```python
from build123d import *

# Parameters (mm, degrees)
SKETCH2_W               = 26
SKETCH2_H               = 26
BOSS_EXTRUDE1_DEPTH     = 53
CUT_EXTRUDE2_DEPTH      = 1
CUT_EXTRUDE2_DEPTH_BACK = 54
SKETCH4_W               = 11
SKETCH4_H               = 5
CUT_EXTRUDE3_DEPTH      = 27
SKETCH5_W               = 17
SKETCH5_H               = 17
CUT_EXTRUDE4_DEPTH      = 21.226470685
BOSS_EXTRUDE3_DEPTH     = 7
BOSS_EXTRUDE4_DEPTH     = 7


with BuildPart() as part:
    # Sketch2 → Boss-Extrude1 (new body)
    with BuildSketch(Plane(origin=(0, 0, 0), x_dir=(0, 0, -1), z_dir=(1, 0, 0))):
        with Locations((13, 13)):
            Rectangle(SKETCH2_W, SKETCH2_H)
    extrude(amount=BOSS_EXTRUDE1_DEPTH)

    # Sketch3 → Cut-Extrude2 (cut, two sides)
    with BuildSketch(Plane(origin=(53, 0, 0), x_dir=(0, 0, -1), z_dir=(1, 0, 0))) as cut_extrude2_sk:
        Polygon((-52.490719717, -64.988510126), (0, 0), (21, 26), (73.490719717, 90.988510126), (-56.486300535, 195.969949561), (-182.46773997, 39.992929308), align=None)
    extrude(amount=CUT_EXTRUDE2_DEPTH, mode=Mode.SUBTRACT)
    extrude(cut_extrude2_sk.sketch, amount=-CUT_EXTRUDE2_DEPTH_BACK, mode=Mode.SUBTRACT)

    # Sketch4 → Cut-Extrude3 (cut, through all)
    with BuildSketch(Plane(origin=(0, 0, -26), x_dir=(-1, 0, 0), z_dir=(0, 0, -1))):
        with Locations((-5.5, 23.5)):
            Rectangle(SKETCH4_W, SKETCH4_H)
        with Locations((-47.5, 23.5)):
            Rectangle(SKETCH4_W, SKETCH4_H)
    extrude(amount=-CUT_EXTRUDE3_DEPTH, mode=Mode.SUBTRACT)

    # Sketch5 → Cut-Extrude4 (cut, through all)
    with BuildSketch(Plane(origin=(0, 0, 0), x_dir=(1, 0, 0), z_dir=(0, 0.628337107, 0.77794118))):
        with Locations((26.5, 15.5)):
            Rectangle(SKETCH5_W, SKETCH5_H)
    extrude(amount=-CUT_EXTRUDE4_DEPTH, mode=Mode.SUBTRACT)

    # Sketch6 → Boss-Extrude3 (add)
    with BuildSketch(Plane(origin=(53, 0, 0), x_dir=(0, 0, -1), z_dir=(1, 0, 0))):
        Polygon((0, 0), (0, 16.7), (13.488461538, 16.7), align=None)
    extrude(amount=-BOSS_EXTRUDE3_DEPTH)

    # Sketch8 → Boss-Extrude4 (add)
    with BuildSketch(Plane.ZY):
        Polygon((0, 0), (0, 16.7), (-13.488461538, 16.7), align=None)
    extrude(amount=-BOSS_EXTRUDE4_DEPTH)


solid = part.part
```
The model under review builds one solid part; all positions refer to its coordinate system, in mm. A direction names the side the tool comes from. Give positions to 0.01 mm unless a question says otherwise; leave off trailing zeros. Write each loop counter-clockwise with the first axis right and the second up, starting at its lowest first coordinate (ties: lowest second). Pieces come first, ordered by that corner, then holes.
(1) Consider section D-D, the plane x = 49. Give the boundary of the cut face in (y, z).
(2) The part is to be moulded in two halves that separate along X. For faces 6 (the flat face through (26.381, 2.761, -7.722)), 7 (the flat face through (50, 16.7, -7)), 8 (the flat face through (53, 8, -13)), 9 (the flat face through (7, 12, -4)), say which applies: released by +X, released by -X, zero draft, split by the parting line, or undercut.
(3) Consider section B-B, the plane y = 9. Give the boundary of the cut face in (x, z), and give its area (3 significant figures).
(4) Consider section C-C, the plane z = -2.25. Give the boundary of the cut face in (x, y), and give its area (3 significant figures).
(5) For P1, Ø1.5, axis at y = 23.5, z = -21.5, coming from the -X side; P2, Ø10, axis at x = 4, z = -22.5, coming from the +Y side; P3, Ø3.5, axis at x = 48, z = -9, coming from the +Y side; P4, Ø4, axis at y = 4, z = -7.5, coming from the -X side, all flat-tipped, find the tip position at first contact; note any pin that passes through.
(6) Tool access review of faces 1 (the flat face through (35, 7, -16)), 2 (the flat face through (26.381, 14.322, -20.464)), 3 (the flat face through (3, 16.7, -7)), 4 (the flat face through (48, 21, -22)), 5 (the flat face through (11, 23, -23)): name each direction out of +Z, -Z, +X, -X, +Y, -Y from which nothing blocks a thin tool from reaching the whole face with its end or side.
(7) Consider section A-A, the plane x = 33. Give the boundary of the cut face in (y, z).
(8) To check wall thickness, follow L1, parallel to X at y = 6.5, z = -15.75; L2, parallel to X at y = 14.5, z = -7.25; L3, parallel to X at y = 21.5, z = -24.25. State the ranges of each line that lie inside material, in increasing order.
Returned:
1. outline: (0, -26) - (21, -26) - (21, -16.96) - (16.7, -13.49) - (16.7, 0) - (0, 0) - close
2. face 6: undercut
2. face 7: zero draft
2. face 8: released by +X
2. face 9: undercut
3. outline: (0, -26) - (18, -26) - (18, -7.27) - (7, -7.27) - (7, 0) - (0, 0) - close; (35, -26) - (53, -26) - (53, 0) - (46, 0) - (46, -7.27) - (35, -7.27) - close
3. area: 776 mm2
4. outline: (0, 0) - (53, 0) - (53, 16.7) - (46, 16.7) - (46, 2.79) - (7, 2.79) - (7, 16.7) - (0, 16.7) - close
4. area: 342 mm2
5. P1: stops at x = 11
5. P2: stops at y = 21
5. P3: stops at y = 16.7
5. P4: stops at x = 0
6. face 1: none
6. face 2: +Z, -Y
6. face 3: +Z, +X, -X, +Y
6. face 4: +Z, -Z, +X, +Y
6. face 5: +Z, -Z, -X, +Y
7. outline: (0, -11.14) - (5.45, -4.4) - (0, 0) - close; (9.85, -26) - (26, -26) - (26, -21) - (18.67, -15.08) - close
8. L1: x = 0 to 18, 35 to 53
8. L2: x = 0 to 7, 46 to 53
8. L3: x = 11 to 42
